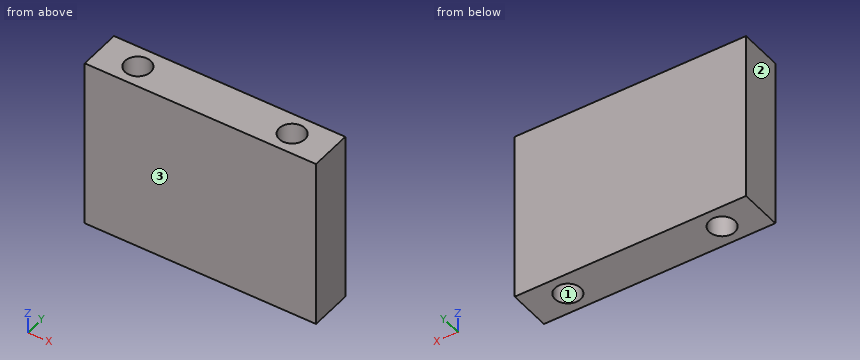
```python
from build123d import *

# Parameters (mm, degrees)
SKETCH1_W               = 27
SKETCH1_H               = 20
BOSS_EXTRUDE1_DEPTH     = 5
SKETCH2_R               = 1.5
CUT_EXTRUDE1_DEPTH      = 1000
CUT_EXTRUDE1_DEPTH_BACK = 1000


with BuildPart() as part:
    # Sketch1 → Boss-Extrude1 (new body)
    with BuildSketch(Plane(origin=(0, 0, 0), x_dir=(1, 0, 0), z_dir=(0, 1, 0))):
        with Locations((13.5, 10)):
            Rectangle(SKETCH1_W, SKETCH1_H)
    extrude(amount=BOSS_EXTRUDE1_DEPTH)

    # Sketch2 → Cut-Extrude1 (cut, two sides)
    with BuildSketch(Plane.XY) as cut_extrude1_sk:
        with Locations((4.5, 2.5)):
            Circle(SKETCH2_R)
        with Locations((22.5, 2.5)):
            Circle(SKETCH2_R)
    extrude(amount=CUT_EXTRUDE1_DEPTH, mode=Mode.SUBTRACT)
    extrude(cut_extrude1_sk.sketch, amount=-CUT_EXTRUDE1_DEPTH_BACK, mode=Mode.SUBTRACT)


solid = part.part
```
The model under review builds one solid part; all positions refer to its coordinate system, in mm. Face numbers are marked on the shaded views. Give positions to 0.01 mm unless a question says otherwise; leave off trailing zeros. Write each loop counter-clockwise with the first axis right and the second up, starting at its lowest first coordinate (ties: lowest second). Pieces come first, ordered by that corner, then holes. Notation, with made-up numbers: M -13.75,-1 L -3.75,-1 A34 ccw -3.75,29 Z; hole C 76,-11.75 d4. An arc over 180 degrees is marked long. Write each question's results on one line, items separated by ' | '. Start each with the question number.
1. For probe 1 along Y at (x, z) = (22.5, -14.5); probe 2 along X at (y, z) = (2.9, -15.75); probe 3 along X at (y, z) = (1.4, -7), list the stretches that pass through material, from the lowest coordinate up. Write a range as [from, to].
2. We need section C-C (z = -13.75). Write out the cut boundary in (x, y).
3. Insertion check: pin 1 Ø12 at (x, z) = (16.5, -16.5) entering from -Y. The pin has a flat end and moves straight along its axis. Give the tip position at first contact, or say it passes through.
4. Mouldability with a two-part tool opening along X and no side actions: class the marked faces 1, 2 and 3 as released by +X, released by -X, zero draft, split by the parting line, or undercut.
5. We need section A-A (x = 22.5). Write out the cut boundary in (y, z), and give its area (3 significant figures).
6. We need section B-B (y = 2.5). Write out the cut boundary in (x, z), and give its area (3 significant figures).
Results found:
1) probe 1: y = [0, 1], [4, 5] | probe 2: x = [0, 3.05], [5.95, 21.05], [23.95, 27] | probe 3: x = [0, 3.48], [5.52, 21.48], [23.52, 27]
2) outline: M 0,0 L 27,0 L 27,5 L 0,5 Z; hole C 4.5,2.5 d3; hole C 22.5,2.5 d3
3) pin 1: stops at y = 0
4) face 1: undercut | face 2: released by -X | face 3: zero draft
5) outline: M 0,-20 L 1,-20 L 1,0 L 0,0 Z; M 4,-20 L 5,-20 L 5,0 L 4,0 Z | area: 40.0 mm^2
6) outline: M 0,-20 L 3,-20 L 3,0 L 0,0 Z; M 6,-20 L 21,-20 L 21,0 L 6,0 Z; M 24,-20 L 27,-20 L 27,0 L 24,0 Z | area: 420 mm^2
